Can you work these out from the model? Positions are in its coordinate system, mm. Coordinates: 2 decimals unless noted, no trailing zeros. Order: outer loops, then holes, each group sorted by start corner. A loop starts at its lowest first (then second) coordinate and runs counter-clockwise, first axis right, second up. Notation, with made-up numbers: (81.5, 68.5) - (96.5, 68.5) arc R24 cw to (96.5, 100.5) - close; hole circle Ø3 at (5.5, 57.25). An arc over 180 degrees is marked (long way). Use a Markdown table: item, result. Add a question column.
(1) We'd pull the mould along X, two halves only. Please class faces 1 (the cylindrical face through (-8.796, 199.903, 3.944)), 2 (the cylindrical face through (-8.14, 169.91, 3.94)), 3 (the flat face through (-2, 178, 0)): pulls with the +X half, pulls with the -X half, needs draft (parallel to the pull), parting line crosses it, or undercut.
(2) I want a section at C-C (x = 0). List the corners of the cut face in (y, z) for me, and give its area (3 significant figures).
(3) I want a section at B-B (z = 3.5). List the corners of the cut face in (x, y) for me.
(4) I want a section at A-A (y = -70). List the corners of the cut face in (x, z) for me, and give its area (3 significant figures).
(5) I want a section at D-D (y = -156). List the corners of the cut face in (x, z) for me, and give its area (3 significant figures).
(6) If I drill on L1, parallel to X at y = -100.5, z = 3; L2, parallel to X at y = -6.5, z = 6.5; L3, parallel to X at y = -182.5, z = 5, over which ranges is the centre line in solid material (lowest first)? Write a range as [from, to].
(7) For pin 1 Ø3 at (y, z) = (-39, 1) entering from +X; pin 2 Ø3 at (y, z) = (-27, 3) entering from -X; pin 3 Ø2.5 at (x, z) = (395, 5) entering from -Y, each with a flat end and sliding along its axis, tell me the tip position at first contact or that it passes through.
Autodesk Inventor part; units mm, degrees
ref_plane "YZ Plane" through (0, 0, 0) normal (1, 0, 0) x (0, 1, 0)
ref_plane "XZ Plane" through (0, 0, 0) normal (0, 1, 0) x (-1, 0, 0)
ref_plane "XY Plane" through (0, 0, 0) normal (0, 0, 1) x (1, 0, 0)
ref_plane "Work Plane1" through (0, 0, 0) normal (0, 0, 1) x (1, 0, 0)
sketch "Sketch1" plane through (0, 0, 0) normal (0, 0, 1) x (1, 0, 0)
  line L0 (250, -200) -> (400, -200) construction
  arc A0 (400, -200) -> (-400, -200) centre (0, -200) ccw construction
  line L1 (-400, -200) -> (-250, -200) construction
  arc A1 (250, -200) -> (-250, -200) centre (0, -200) ccw construction
  arc A2 (400, -200) -> (-400, -200) centre (0, -200) ccw
  arc A3 (370, -200) -> (-370, -200) centre (0, -200) ccw
  line L2 (400, -200) -> (370, -200) construction
  line L3 (385, -200) -> (385, -231.622) construction
  arc A4 (385, -222.5) -> (388.75, -208.5048) centre (385, -215) ccw
  line L4 (388.75, -208.5048) -> (388.75, -200)
  line L5 (400, -200) -> (388.75, -200)
  arc A5 (381.25, -208.5048) -> (385, -222.5) centre (385, -215) ccw
  line L6 (381.25, -208.5048) -> (381.25, -200)
  line L7 (370, -200) -> (381.25, -200)
  line L8 (-381.25, -191.4952) -> (-381.25, -200)
  arc A6 (-381.25, -191.4952) -> (-385, -177.5) centre (-385, -185) ccw
  line L9 (-370, -200) -> (-381.25, -200)
  arc A7 (-385, -177.5) -> (-388.75, -191.4952) centre (-385, -185) ccw
  line L10 (-388.75, -191.4952) -> (-388.75, -200)
  line L11 (-400, -200) -> (-388.75, -200)
  point P0 (0, 0)
  point P1 (-400, -200)
  point P2 (-370, -200)
  dimension "d0" = 30
  dimension "d1" = 7.5
  dimension "d2" = 7.5
  dimension "d3" = 15
  dimension "d6" = 180
extrude "Extrusion1" add sketch "Sketch1" along normal blind 8
properties part number "barrier"
Answers follow:
| question | item | result |
|---|---|---|
| 1 | face 1 | parting line crosses it |
| 1 | face 2 | undercut |
| 1 | face 3 | needs draft |
| 2 | outline | (170, 0) - (200, 0) - (200, 8) - (170, 8) - close |
| 2 | area | 240 mm² |
| 3 | outline | (-400, -200) - (-388.75, -200) - (-388.75, -191.5) arc R7.5 cw to (-385, -177.5) arc R7.5 cw to (-381.25, -191.5) - (-381.25, -200) - (-370, -200) arc R370 cw to (370, -200) - (381.25, -200) - (381.25, -208.5) arc R7.5 ccw to (385, -222.5) arc R7.5 ccw to (388.75, -208.5) - (388.75, -200) - (400, -200) arc R400 ccw to start |
| 4 | outline | (-378.29, 0) - (-346.41, 0) - (-346.41, 8) - (-378.29, 8) - close; (346.41, 0) - (378.29, 0) - (378.29, 8) - (346.41, 8) - close |
| 4 | area | 510 mm² |
| 5 | outline | (-397.57, 0) - (-367.37, 0) - (-367.37, 8) - (-397.57, 8) - close; (367.37, 0) - (397.57, 0) - (397.57, 8) - (367.37, 8) - close |
| 5 | area | 483 mm² |
| 6 | L1 | x = [-387.43, -356.37], [356.37, 387.43] |
| 6 | L2 | x = [-350.08, -315.37], [315.37, 350.08] |
| 6 | L3 | x = [-399.62, -392.07], [-377.93, -369.59], [369.59, 399.62] |
| 7 | pin 1 | stops at x = 366.82 |
| 7 | pin 2 | stops at x = -361.37 |
| 7 | pin 3 | stops at y = -200 |
